Design review of the part built by this model. Coordinates are the model's own, in mm. Face numbers are marked on the shaded views. A direction names the side the tool comes from. Round coordinates to 2 decimals unless told otherwise and drop trailing zeros. Order: outer loops, then holes, each group sorted by start corner. A loop starts at its lowest first (then second) coordinate and runs counter-clockwise, first axis right, second up. Notation, with made-up numbers: M 2,-21 L 49,-21 A28 ccw 49,9 Z; hole C 77.5,81 d7. An arc over 180 degrees is marked long. Use a Markdown table: item, result. Add a question column.
(1) To check wall thickness, follow probe 1 along Y at (x, z) = (-11, 2.5); probe 2 along Y at (x, z) = (5.5, 0.5); probe 3 along X at (y, z) = (-8.75, -9.5). State the ranges of each line that lie inside material, in increasing order. Write a range as from..to.
(2) Take a section at B-B (x = 8). Write out the cut boundary in (y, z).
(3) For pin 1 (7.5 mm diameter, centred on x = 3.5, z = -15.5, fed in from -Y); pin 2 (5 mm diameter, centred on x = 9.5, z = 3, fed in from -Y); pin 3 (19.5 mm diameter, centred on x = -8.5, z = -10.5, fed in from -Y), all flat-tipped, find the tip position at first contact; note any pin that passes through.
(4) Take a section at C-C (y = -7). Write out the cut boundary in (x, z).
(5) Take a section at D-D (y = -17.5). Write out the cut boundary in (x, z).
(6) Machinability: for the marked faces 1, 2 and 3, which of the approach directions +Z, -Z, +X, -X, +Y, -Y give a long, thin tool a straight path to every point of the face, cutting with its end or side? Answer none if there is none.
(7) Take a section at A-A (z = 20.5). Write out the cut boundary in (x, y), then the cut area to 3 significant figures.
(8) The part is to be moulded in two halves that separate along X. For the marked faces 4, 5 and 6, say which applies: released by +X, released by -X, zero draft, split by the parting line, or undercut.
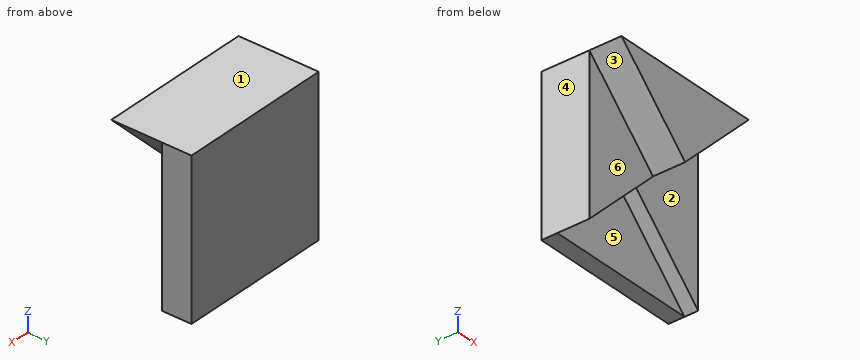
```python
from build123d import *

# Parameters (mm, degrees)
F1_DEPTH = 25.4
F2_DEPTH = 15.24
F3_DEPTH = 9.398
F4_DEPTH = 5.08


with BuildPart() as f1:
    # F0 (on Front) → F1 (new body)
    with BuildSketch(Plane.XZ):
        Polygon((0, 0), (24.510982, 24.510982), (-24.510982, 24.510982), align=None)
    extrude(amount=F1_DEPTH)

    # F0 (on Front) → F2 (join)
    with BuildSketch(Plane.XZ):
        Polygon((-24.510982, 24.510982), (-24.510982, -24.510982), (0, 0), align=None)
    extrude(amount=F2_DEPTH)

    # F0 (on Front) → F3 (join)
    with BuildSketch(Plane.XZ):
        Polygon((0, 0), (24.510982, -24.510982), (24.510982, 24.510982), align=None)
    extrude(amount=F3_DEPTH)

    # F0 (on Front) → F4 (join)
    with BuildSketch(Plane.XZ):
        Polygon((-24.510982, -24.510982), (24.510982, -24.510982), (0, 0), align=None)
    extrude(amount=F4_DEPTH)


solid = f1.part
```
Verdict:
| question | item | result |
|---|---|---|
| 1 | probe 1 | y = -15.24..0 |
| 1 | probe 2 | y = -9.4..0 |
| 1 | probe 3 | x = -24.51..-9.5, 9.5..24.51 |
| 2 | outline | M -25.4,8 L -9.4,8 L -9.4,-8 L -5.08,-8 L -5.08,-24.51 L 0,-24.51 L 0,24.51 L -25.4,24.51 Z |
| 3 | pin 1 | stops at y = -5.08 |
| 3 | pin 2 | stops at y = -9.4 |
| 3 | pin 3 | stops at y = -15.24 |
| 4 | outline | M -24.51,-24.51 L 0,0 L 24.51,-24.51 L 24.51,24.51 L -24.51,24.51 Z |
| 5 | outline | M -24.51,24.51 L 0,0 L 24.51,24.51 Z |
| 6 | face 1 | +Z, +X, -X, +Y, -Y |
| 6 | face 2 | -Z, +X, -Y |
| 6 | face 3 | -Z, -X, -Y |
| 7 | outline | M -24.51,-15.24 L -20.5,-15.24 L -20.5,-25.4 L 20.5,-25.4 L 20.5,-9.4 L 24.51,-9.4 L 24.51,0 L -24.51,0 Z |
| 7 | area | 1,140 mm^2 |
| 8 | face 4 | released by -X |
| 8 | face 5 | undercut |
| 8 | face 6 | zero draft |
